Part model, mm, in its own coordinate system. A direction names the side the tool comes from. Round coordinates to 2 decimals unless told otherwise and drop trailing zeros. Write each loop counter-clockwise with the first axis right and the second up, starting at its lowest first coordinate (ties: lowest second). Pieces come first, ordered by that corner, then holes.
1) Saw through at A-A on z = -12.75. Write the cut outline in (x, y).
2) Saw through at C-C on z = -2.75. Write the cut outline in (x, y), and give its area (3 significant figures).
3) Flat gauge pins, fed straight in: pin 1 (2 mm diameter, centred on x = -1, y = -43.5, fed in from -Z); pin 2 (0.8 mm diameter, centred on y = -22, z = 1.5, fed in from +X); pin 3 (1.9 mm diameter, centred on x = -5.5, y = -40.5, fed in from -Z); pin 4 (4 mm diameter, centred on x = -2.5, z = 1, fed in from +Y). Where does each tip first touch, or does it go through?
4) Pull direction X, two halves, no side cores. Call faces 1 (the flat face through (5.627, -41.905, 5.726)), 2 (the flat face through (-7.525, -42, 3)), 3 (the flat face through (0, -42, 7.5)), 4 (the cylindrical face through (17.124, -82.972, -8.498)): +X half, -X half, draft (parallel to the pull), parting line (faces both ways), or undercut.
5) Drill centre lines: L1, parallel to Y at x = -13, z = -3; L2, parallel to Z at x = 3, y = -47; L3, parallel to X at y = -34.5, z = 3.25. Where is each one in solid material? Low to high.
6) Which spindle directions (+Z, -Z, +X, -X, +Y, -Y) get a long thin tool onto all of the face, cutting with end or side? Do faces 5 (the cylindrical face through (-0.175, -82.972, -8.643)), 6 (the flat face through (0, -40, 0)), 7 (the flat face through (11, -83, 0)). Say none if no direction does.
7) Saw through at D-D on x = 0.5. Write the cut outline in (y, z), and give its area (3 significant figures).
8) Saw through at B-B on y = -70.5. Write the cut outline in (x, z), and give its area (3 significant figures).
```python
from build123d import *

# Parameters (mm, degrees)
F1_DEPTH = 85
F2_W     = 35
F2_H     = 15
F3_DEPTH = 4
F5_D     = 3.3
F5_DEPTH = 30
F5_TIP   = 0.9914200214
F7_D     = 22
F7_DEPTH = 30
F7_TIP   = 6.6094668093


with BuildPart() as f1:
    # F0 (on Front) → F1 (new body)
    with BuildSketch(Plane.XZ):
        Polygon((-3.7746716016, 2.5), (-3.7746716016, 0), (3.7253283984, 0), (3.7253283984, 2.5), (7.4753283984, 2.5), (7.4753283984, 4), (3.7253283984, 7.5), (-3.7746716016, 7.5), (-7.5246716016, 4), (-7.5246716016, 2.5), align=None)
    extrude(amount=F1_DEPTH)

    # F2 (on face) → F3 (join)
    with BuildSketch(Plane.XZ.offset(85)):
        with Locations((-0.0246716016, -7.5)):
            Rectangle(F2_W, F2_H)
    extrude(amount=-F3_DEPTH)

    # F5
    with Locations(Plane.XZ.offset(85)):
        with Locations((-15.5246716016, -9), (15.4753283984, -8.5702965236)):
            Hole(F5_D / 2, depth=F5_DEPTH)
            with Locations((0, 0, -(F5_DEPTH + F5_TIP / 2))):  # 118° drill point
                Cone(0, F5_D / 2, F5_TIP, mode=Mode.SUBTRACT)

    # F7
    with Locations(Plane.XZ.offset(85)):
        with Locations((0, -19.6417048573)):
            Hole(F7_D / 2, depth=F7_DEPTH)
            with Locations((0, 0, -(F7_DEPTH + F7_TIP / 2))):  # 118° drill point
                Cone(0, F7_D / 2, F7_TIP, mode=Mode.SUBTRACT)


solid = f1.part
```
Completed:
1. outline: (-17.52, -85) - (-8.57, -85) - (-8.57, -81) - (-17.52, -81) - close; (8.57, -85) - (17.48, -85) - (17.48, -81) - (8.57, -81) - close
2. outline: (-17.52, -85) - (17.48, -85) - (17.48, -81) - (-17.52, -81) - close
2. area: 140 mm2
3. pin 1: stops at z = 0
3. pin 2: stops at x = 3.73
3. pin 3: stops at z = 2.5
3. pin 4: stops at y = 0
4. face 1: +X half
4. face 2: -X half
4. face 3: draft
4. face 4: undercut
5. L1: y = -85 to -81
5. L2: z = 0 to 7.5
5. L3: x = -7.52 to 7.48
6. face 5: -Z, +Y, -Y
6. face 6: -Z, +X, -X, +Y
6. face 7: +X, +Y, -Y
7. outline: (-85, -8.65) - (-81, -8.65) - (-81, 0) - (0, 0) - (0, 7.5) - (-85, 7.5) - close
7. area: 672 mm2
8. outline: (-7.52, 2.5) - (-3.77, 2.5) - (-3.77, 0) - (3.73, 0) - (3.73, 2.5) - (7.48, 2.5) - (7.48, 4) - (3.73, 7.5) - (-3.77, 7.5) - (-7.52, 4) - close
8. area: 80.6 mm2
